Part model, mm, in its own coordinate system. A direction names the side the tool comes from. Give positions to 0.01 mm unless a question says otherwise; leave off trailing zeros. Write each loop counter-clockwise with the first axis right and the second up, starting at its lowest first coordinate (ties: lowest second). Pieces come first, ordered by that corner, then holes.
```python
from build123d import *

# Parameters (mm, degrees)
SKETCH1_W           = 25.4
SKETCH1_H           = 25.4
BOSS_EXTRUDE1_DEPTH = 3
SKETCH2_R           = 5
BOSS_EXTRUDE2_DEPTH = 40
CHAMFER1_SIZE       = 10


with BuildPart() as part:
    # Sketch1 → Boss-Extrude1 (new body)
    with BuildSketch(Plane(origin=(0, 0, 0), x_dir=(1, 0, 0), z_dir=(0, 1, 0))):
        Rectangle(SKETCH1_W, SKETCH1_H)
    extrude(amount=BOSS_EXTRUDE1_DEPTH)

    # Sketch2 → Boss-Extrude2 (add)
    with BuildSketch(Plane(origin=(0, 3, 0), x_dir=(1, 0, 0), z_dir=(0, 1, 0))):
        with Locations(Location((0, 0, 0), (0, 0, 270))):
            Circle(SKETCH2_R)
    extrude(amount=BOSS_EXTRUDE2_DEPTH)

    # Chamfer1
    # the kernel refuses this chamfer: 10 mm, written as the material it adds along each edge
    with BuildSketch(Plane(origin=(0, 3, 0), x_dir=(0, 0, 1), z_dir=(-1, 0, 0))) as chamfer1_piece_1_section:
        Polygon((5 + CHAMFER1_SIZE, 0), (5, CHAMFER1_SIZE), (5, 0), align=None)
    chamfer1_piece_1 = revolve(axis=Axis((0, 3, 0), (0, 1, 0)), mode=Mode.PRIVATE)
    chamfer1_piece_1 = split(chamfer1_piece_1, bisect_by=Plane(origin=(0, 7.901138133, -12.7), z_dir=(0, 0, 1)), keep=Keep.TOP, mode=Mode.PRIVATE)
    chamfer1_piece_1 = split(chamfer1_piece_1, bisect_by=Plane(origin=(-12.7, 7.901138133, -9.901138133), z_dir=(1, 0, 0)), keep=Keep.TOP, mode=Mode.PRIVATE)
    chamfer1_piece_1 = split(chamfer1_piece_1, bisect_by=Plane(origin=(12.7, 7.901138133, -9.901138133), z_dir=(-1, 0, 0)), keep=Keep.TOP, mode=Mode.PRIVATE)
    chamfer1_piece_1 = split(chamfer1_piece_1, bisect_by=Plane(origin=(0, 7.901138133, 12.7), z_dir=(0, 0, -1)), keep=Keep.TOP, mode=Mode.PRIVATE)
    add(chamfer1_piece_1)

    # Sketch3 → Revolve1 (revolve)
    with BuildSketch(Plane(origin=(0, 0, 0), x_dir=(0, 0, -1), z_dir=(1, 0, 0)), mode=Mode.PRIVATE) as revolve1_sk:
        Polygon((0, 55), (0, 43), (5, 43), align=None)
    revolve(revolve1_sk.sketch.rotate(Axis((0, 0, 0), (0, 1, 0)), 327.850947574), axis=Axis((0, 0, 0), (0, 1, 0)))


solid = part.part
```
1) Saw through at C-C, the plane y = 49. Write the cut outline in (x, z).
Answers follow:
outline: circle Ø5 at (0, 0)
2) Saw through at A-A, the plane y = 4.5. Write the cut outline in (x, z).
Answers follow:
outline: (-12.7, -4.58) arc R13.5 ccw to (-4.58, -12.7) - (4.58, -12.7) arc R13.5 ccw to (12.7, -4.58) - (12.7, 4.58) arc R13.5 ccw to (4.58, 12.7) - (-4.58, 12.7) arc R13.5 ccw to (-12.7, 4.58) - close
3) Pin check, flat tips, straight feed: pin 1 Ø4 at (x, z) = (9.5, -9.5) entering from +Y (3 decimals); pin 2 Ø1 at (x, y) = (2.5, 24) entering from -Z; pin 3 Ø6 at (y, z) = (12, 5.5) entering from -X; pin 4 Ø2 at (x, y) = (7, 32.5) entering from +Z. Stop position of each tip, or through.
Answers follow:
pin 1: stops at y = 6.565
pin 2: stops at z = -4.58
pin 3: stops at x = -7.62
pin 4: passes through
4) 3-axis set-ups, long thin cutter, end or side, ignore diameter. For faces 1 (the face through (-11, 3, 11)), 2 (the face through (-4.88, 27.79, -1.08)), 3 (the face through (11, 3, -11)), 4 (the face through (11, 3, 11)), 5 (the face through (-11, 3, -11)): which of +Z, -Z, +X, -X, +Y, -Y reach the whole face in a straight line?
Answers follow:
face 1: +Z, -X, +Y
face 2: +Y
face 3: -Z, +X, +Y
face 4: +Z, +X, +Y
face 5: -Z, -X, +Y
5) Wall check: L1, parallel to X at y = 13, z = -0.25; L2, parallel to Y at x = -0.5, z = -10; L3, parallel to X at y = 7, z = 6.5. Give the ranges that are in metal, low to high.
Answers follow:
L1: x = -4.99 to 4.99
L2: y = 0 to 7.99
L3: x = -8.87 to 8.87
6) Saw through at B-B, the plane y = 38.5. Write the cut outline in (x, z).
Answers follow:
outline: circle Ø10 at (0, 0)
